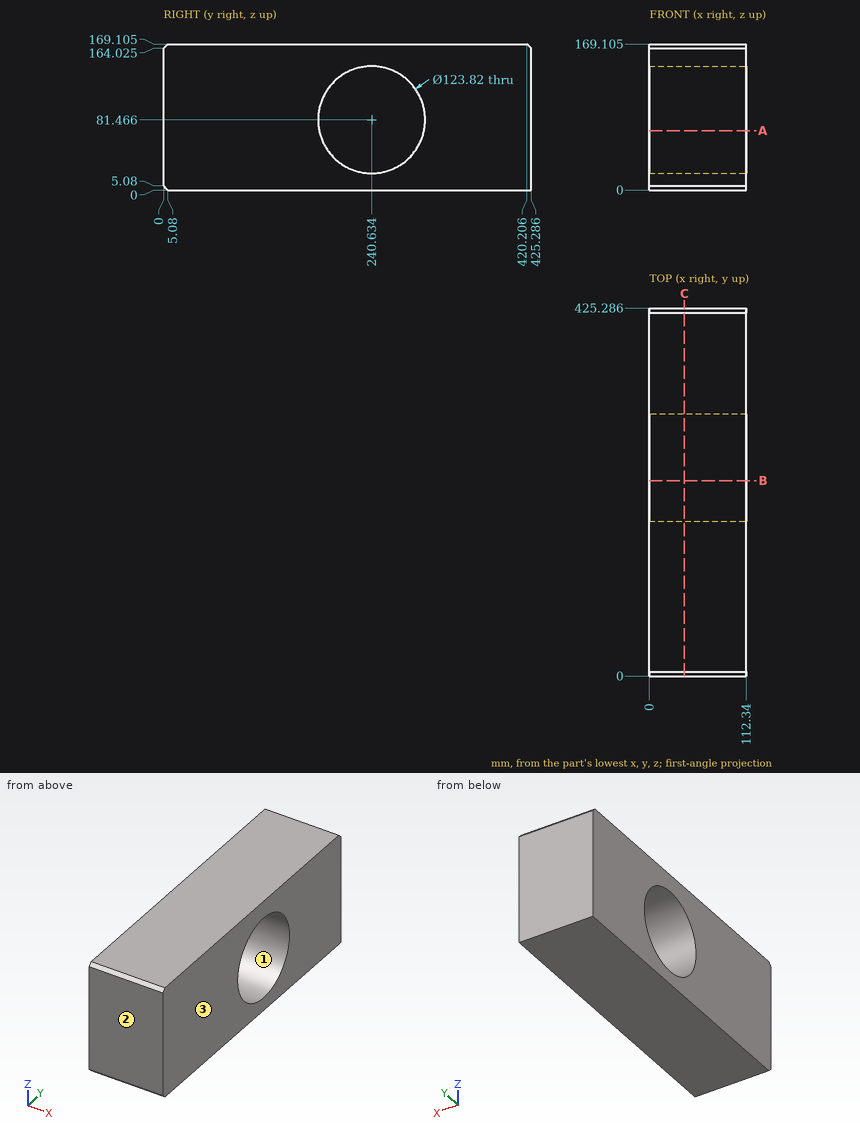
For this review, use the dimensioned drawing (mm, ordinates from the lowest corner) and the shaded views. Give positions to 0.01 mm unless a question says otherwise; leave off trailing zeros. Order: outer loops, then holes, each group sorted by start corner. A loop starts at its lowest first (then second) coordinate and runs counter-clockwise, first axis right, second up. Notation, with made-up numbers: (7, -7.5) - (20, -7.5) arc R30 cw to (20, 19.5) - close; hole circle Ø9 at (59.5, 15.5). An arc over 180 degrees is marked (long way). Use CSV: the item, a comma, the result in double quotes. Start each with the question number.
Q1. We need section C-C, the plane x = 40.5. Write out the cut boundary in (y, z) (1 decimal), and give its area (3 significant figures).
Q2. The part is to be moulded in two halves that separate along Y. For the marked faces 1, 2 and 3, say which applies: +Y half, -Y half, draft (parallel to the pull), parting line (faces both ways), or undercut.
Q3. To check wall thickness, follow line 1 along Z through (x, y) = (82, 185) (1 decimal); line 2 along Y through (x, z) = (91, 33) (1 decimal); line 3 along Y through (x, z) = (91, 132.5) (1 decimal). State the ranges of each line that lie inside material, in increasing order. Write a range as [from, to].
Q4. We need section B-B, the plane y = 226. Write out the cut boundary in (x, z) (1 decimal).
Q5. We need section A-A, the plane z = 69. Write out the cut boundary in (x, y) (1 decimal).
Outcome:
1,outline,"(0, 5.1) - (5.1, 0) - (425.3, 0) - (425.3, 164) - (420.2, 169.1) - (5.1, 169.1) - (0, 164) - close; hole circle Ø123.8 at (240.6, 81.5)"
1,area,"59,800 mm^2"
2,face 1,"undercut"
2,face 2,"-Y half"
2,face 3,"draft"
3,line 1,"z = [0, 54.3], [108.6, 169.1]"
3,line 2,"y = [0, 202.1], [279.2, 425.3]"
3,line 3,"y = [0, 205.6], [275.7, 425.3]"
4,outline,"(0, 0) - (112.3, 0) - (112.3, 21.3) - (0, 21.3) - close; (0, 141.6) - (112.3, 141.6) - (112.3, 169.1) - (0, 169.1) - close"
5,outline,"(0, 0) - (112.3, 0) - (112.3, 180) - (0, 180) - close; (0, 301.3) - (112.3, 301.3) - (112.3, 425.3) - (0, 425.3) - close"
